Drawing for the job (mm, zero at the part's lowest x, y, z). Round coordinates to 2 decimals unless told otherwise and drop trailing zeros. Write each loop counter-clockwise with the first axis right and the second up, starting at its lowest first coordinate (ties: lowest second). Pieces come first, ordered by that corner, then holes.
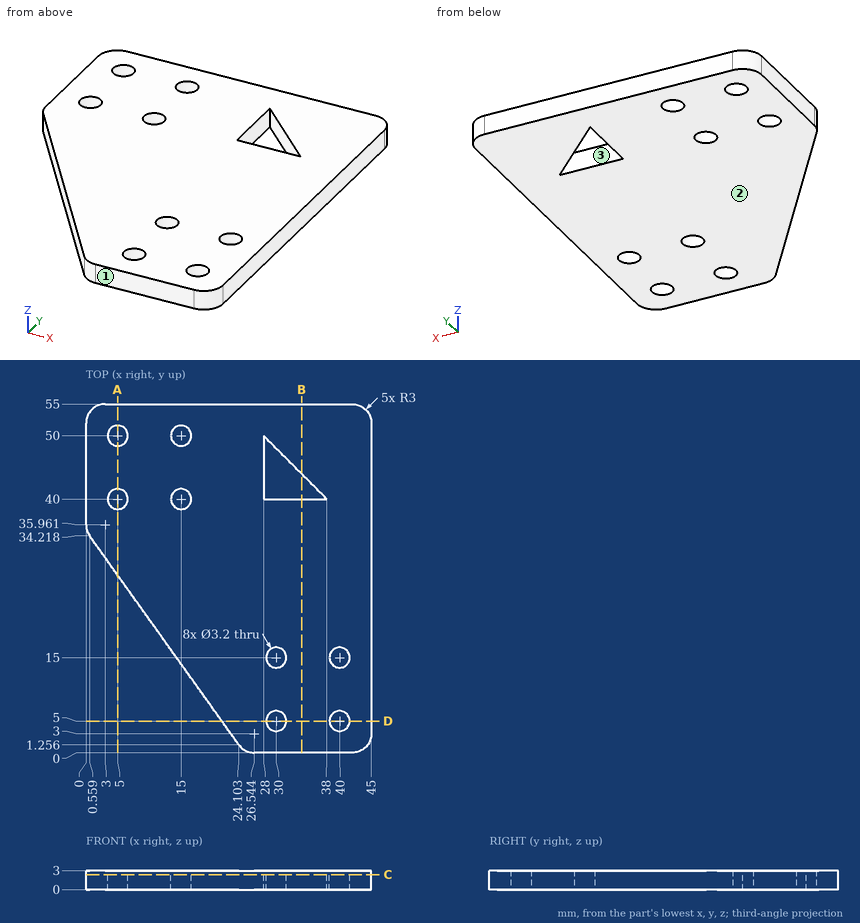
1) Cut at B-B on x = 34. List the corners of the cut face in (y, z).
2) Pull direction Y, two halves, no side cores. Call the marked faces 1, 2 and 3: released by +Y, released by -Y, zero draft, split by the parting line, or undercut.
3) Wall check: probe 1 along Y at (x, z) = (5, 1.75); probe 2 along Y at (x, z) = (40, 2); probe 3 along X at (y, z) = (44, 0.6). Give the ranges that are in metal, low to high.
4) Cut at D-D on y = 5. List the corners of the cut face in (x, z).
5) Flat gauge pins, fed straight in: pin 1 Ø8 at (x, y) = (31, 49.5) entering from -Z; pin 2 Ø1.5 at (y, z) = (16.5, 1) entering from -X; pin 3 Ø2.5 at (x, y) = (15, 50) entering from -Z. Where does each tip first touch, or does it go through?
6) Cut at C-C on z = 2.4. Give the number of separate pieces and of enclosed holes in the cut face, and give its area (3 significant figures).
7) Cut at A-A on x = 5. List the corners of the cut face in (y, z), and give its area (3 significant figures).
Result sheet:
1. outline: (0, 0) - (40, 0) - (40, 3) - (0, 3) - close; (44, 0) - (55, 0) - (55, 3) - (44, 3) - close
2. face 1: released by -Y
2. face 2: zero draft
2. face 3: undercut
3. probe 1: y = 28 to 38.4, 41.6 to 48.4, 51.6 to 55
3. probe 2: y = 0 to 3.4, 6.6 to 13.4, 16.6 to 55
3. probe 3: x = 0 to 28, 34 to 45
4. outline: (21.43, 0) - (28.4, 0) - (28.4, 3) - (21.43, 3) - close; (31.6, 0) - (38.4, 0) - (38.4, 3) - (31.6, 3) - close; (41.6, 0) - (45, 0) - (45, 3) - (41.6, 3) - close
5. pin 1: stops at z = 0
5. pin 2: stops at x = 12.68
5. pin 3: passes through
6. separate pieces: 1
6. enclosed holes: 9
6. area: 1,920 mm2
7. outline: (28, 0) - (38.4, 0) - (38.4, 3) - (28, 3) - close; (41.6, 0) - (48.4, 0) - (48.4, 3) - (41.6, 3) - close; (51.6, 0) - (55, 0) - (55, 3) - (51.6, 3) - close
7. area: 61.8 mm2
